```python
from build123d import *

# Parameters (mm, degrees)
BOSS_EXTRUDE1_DEPTH = 2
SKETCH4_R           = 2
SKETCH4_R_2         = 1.5
CUT_EXTRUDE1_DEPTH  = 2


with BuildPart() as part:
    # Sketch2 → Boss-Extrude1 (new body)
    with BuildSketch(Plane.XY):
        Polygon((0, 0), (0, 2), (0, 60), (43, 60), (115, 60), (173, 2), (173, 0), align=None)
    extrude(amount=BOSS_EXTRUDE1_DEPTH)

    # Sketch4 → Cut-Extrude1 (cut)
    with BuildSketch(Plane.XY.offset(2)):
        with Locations((20, 13)):
            Circle(SKETCH4_R)
        with Locations((121, 13)):
            Circle(SKETCH4_R)
        with Locations((28.5, 13)):
            Circle(SKETCH4_R_2)
        with Locations((112.5, 13)):
            Circle(SKETCH4_R_2)
        with Locations((129.5, 13)):
            Circle(SKETCH4_R_2)
        with Locations((11.5, 13)):
            Circle(SKETCH4_R_2)
    extrude(amount=-CUT_EXTRUDE1_DEPTH, mode=Mode.SUBTRACT)


solid = part.part
```
Verification items for the finished model (mm, model axes). Round coordinates to 2 decimals unless told otherwise and drop trailing zeros. Write each loop counter-clockwise with the first axis right and the second up, starting at its lowest first coordinate (ties: lowest second). Pieces come first, ordered by that corner, then holes. Notation, with made-up numbers: (44, 14) -> (75, 14) arc R20 cw to (75, 44) -> close; hole circle Ø1 at (28, -21.5). An arc over 180 degrees is marked (long way). Write each question's results on one line, items separated by ' | '. Start each with the question number.
1. Material ranges on probe 1 along Y at (x, z) = (112.5, 1.4); probe 2 along Y at (x, z) = (20, 0.7); probe 3 along Y at (x, z) = (162, 0.4), recorded low to high. Write a range as from..to.
2. Depth check by flat-ended pin: P1, Ø4, axis at x = 11.5, y = 13, coming from the +Z side; P2, Ø3.5, axis at x = 121, y = 13, coming from the -Z side. Enter the tip coordinate at first touch or a pass-through.
3. Cross-section at B-B (y = 13). Enter the section's corners in (x, z).
4. Draft check along X on faces 1 (the flat face through (68, 30, 0)), 2 (the cylindrical face through (128, 13, 1)), 3 (the flat face through (144, 31, 1)). Enter one of: +X half, -X half, draft (parallel to the pull), parting line (faces both ways), or undercut.
5. Cross-section at D-D (x = 20). Enter the section's corners in (y, z), then the cut area to 3 significant figures.
6. Cross-section at C-C (z = 0.3). Enter the section's corners in (x, y), then the cut area to 3 significant figures.
7. Cross-section at A-A (x = 129.5). Enter the section's corners in (y, z).
Solutions:
1) probe 1: y = 0..11.5, 14.5..60 | probe 2: y = 0..11, 15..60 | probe 3: y = 0..13
2) P1: stops at z = 2 | P2: passes through
3) outline: (0, 0) -> (10, 0) -> (10, 2) -> (0, 2) -> close; (13, 0) -> (18, 0) -> (18, 2) -> (13, 2) -> close; (22, 0) -> (27, 0) -> (27, 2) -> (22, 2) -> close; (30, 0) -> (111, 0) -> (111, 2) -> (30, 2) -> close; (114, 0) -> (119, 0) -> (119, 2) -> (114, 2) -> close; (123, 0) -> (128, 0) -> (128, 2) -> (123, 2) -> close; (131, 0) -> (162, 0) -> (162, 2) -> (131, 2) -> close
4) face 1: draft | face 2: undercut | face 3: +X half
5) outline: (0, 0) -> (11, 0) -> (11, 2) -> (0, 2) -> close; (15, 0) -> (60, 0) -> (60, 2) -> (15, 2) -> close | area: 112 mm2
6) outline: (0, 0) -> (173, 0) -> (173, 2) -> (115, 60) -> (0, 60) -> close; hole circle Ø3 at (11.5, 13); hole circle Ø4 at (20, 13); hole circle Ø3 at (28.5, 13); hole circle Ø3 at (112.5, 13); hole circle Ø4 at (121, 13); hole circle Ø3 at (129.5, 13) | area: 8,640 mm2
7) outline: (0, 0) -> (11.5, 0) -> (11.5, 2) -> (0, 2) -> close; (14.5, 0) -> (45.5, 0) -> (45.5, 2) -> (14.5, 2) -> close
